Here's the drawing with two shaded views (mm, measured from the low corner). I have some questions. Coordinates: 2 decimals unless noted, no trailing zeros. Order: outer loops, then holes, each group sorted by start corner. A loop starts at its lowest first (then second) coordinate and runs counter-clockwise, first axis right, second up. Notation, with made-up numbers: (89.5, 9.25) -> (128.5, 9.25) arc R14 ccw to (128.5, 18.25) -> close; hole circle Ø10 at (-40, -30.75). An arc over 180 degrees is marked (long way). Answer in a Markdown table with one row per item. Add a question column.
1. Imagine slicing it at C-C on z = 112.5. Write out the boundary of the cut face in (x, y), plus the area to 3 significant figures.
2. If I drill on line 1 along X through (y, z) = (1.15, 18); line 2 along Z through (x, y) = (16.4, 19.95); line 3 along Y through (x, z) = (17, 170), over which ranges is the centre line in solid material (lowest first)? Write a range as [from, to].
3. Imagine slicing it at B-B on y = 3.75. Write out the boundary of the cut face in (x, z), plus the area to 3 significant figures.
4. Will this pin go through, and if not, where does the flat tip stop? pin 1 (4 mm diameter, centred on x = 43, y = 15, fed in from -Z).
5. Imagine slicing it at A-A on x = 36. Write out the boundary of the cut face in (y, z).
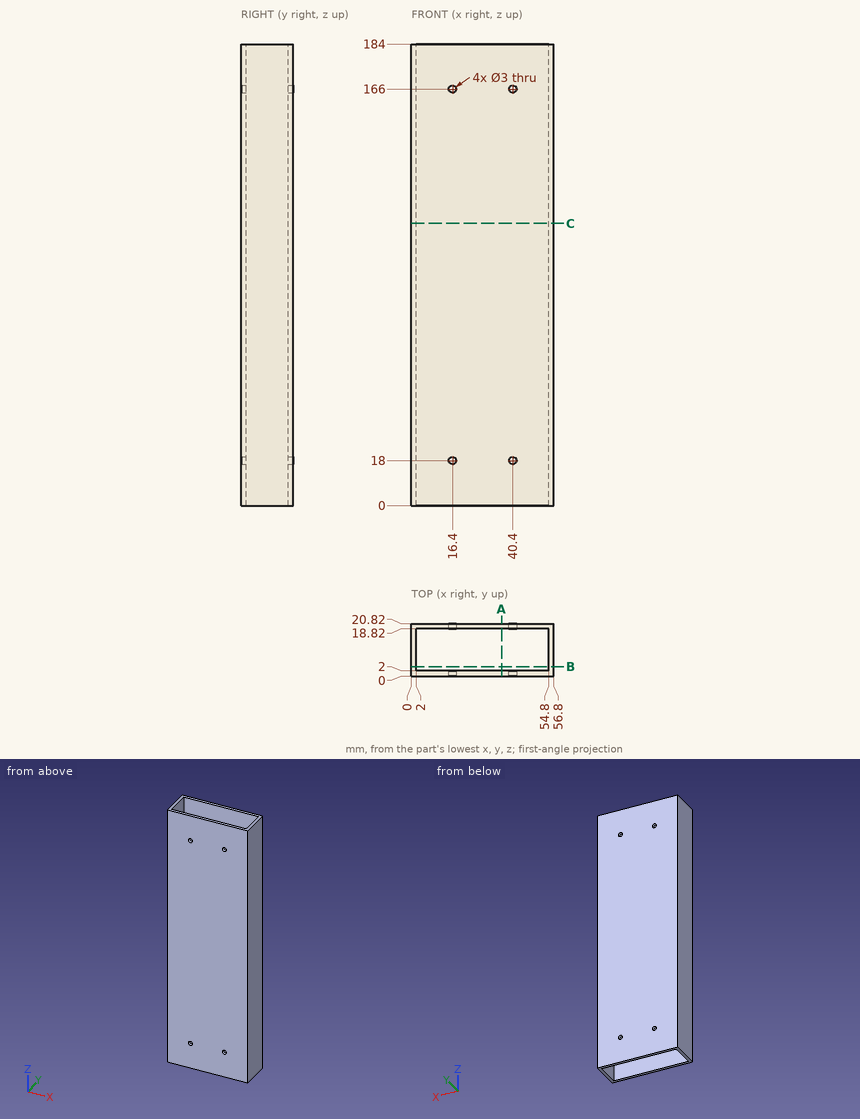
Answers follow:
| question | item | result |
|---|---|---|
| 1 | outline | (0, 0) -> (56.8, 0) -> (56.8, 20.82) -> (0, 20.82) -> close; hole (2, 2) -> (54.8, 2) -> (54.8, 18.82) -> (2, 18.82) -> close |
| 1 | area | 294 mm² |
| 2 | line 1 | x = [0, 14.9], [17.9, 38.9], [41.9, 56.8] |
| 2 | line 2 | z = [0, 16.5], [19.5, 164.5], [167.5, 184] |
| 2 | line 3 | y = [0, 2], [18.82, 20.82] |
| 3 | outline | (0, 0) -> (2, 0) -> (2, 184) -> (0, 184) -> close; (54.8, 0) -> (56.8, 0) -> (56.8, 184) -> (54.8, 184) -> close |
| 3 | area | 736 mm² |
| 4 | pin 1 | passes through |
| 5 | outline | (0, 0) -> (2, 0) -> (2, 184) -> (0, 184) -> close; (18.82, 0) -> (20.82, 0) -> (20.82, 184) -> (18.82, 184) -> close |
